The model under review builds one solid part; all positions refer to its coordinate system, in mm. Face numbers are marked on the shaded views. A direction names the side the tool comes from. Round coordinates to 2 decimals unless told otherwise and drop trailing zeros. Order: outer loops, then holes, each group sorted by start corner. A loop starts at its lowest first (then second) coordinate and runs counter-clockwise, first axis right, second up. Notation, with made-up numbers: (46, 83.5) - (66, 83.5) arc R19 ccw to (66, 118.5) - close; hole circle Ø8 at (10, 64.25). An arc over 180 degrees is marked (long way). One line per question, with ' | ' between items. Start each with the question number.
Item 1: Add section C-C on x = -6.5. State how many separate pieces and enclosed holes the cut face has, and give its area (3 significant figures).
Item 2: Add section B-B on y = 8. State the section outline as (x, z) points.
Item 3: Insertion check: pin 1 Ø5 at (y, z) = (36.5, 5) entering from +X; pin 2 Ø6 at (x, z) = (20.98, -7.33) entering from +Y; pin 3 Ø12 at (x, z) = (14.5, 20) entering from +Y; pin 4 Ø16 at (x, y) = (3.5, 17.5) entering from +Z. Each pin has a flat end and moves straight along its axis. Give the tip position at first contact, or say it passes through.
Item 4: Tool access review of the marked faces 4, 5 and 6: name each direction out of +Z, -Z, +X, -X, +Y, -Y from which nothing blocks a thin tool from reaching the whole face with its end or side.
Item 5: For L1, parallel to Z at x = 0, y = 46; L2, parallel to X at y = 31, z = 4; L3, parallel to Y at x = -2, z = -19.5, list the stretches that pass through material, from the lowest coordinate up. Write a range as [from, to].
Item 6: Add section A-A on y = 49. State the section outline as (x, z) points (1 decimal).
Item 7: Draft analysis for pull direction Z (two halves, no side actions). For the marked faces 1, 2 and 3, state which applies: +Z half, -Z half, draft (parallel to the pull), parting line (faces both ways), or undercut.
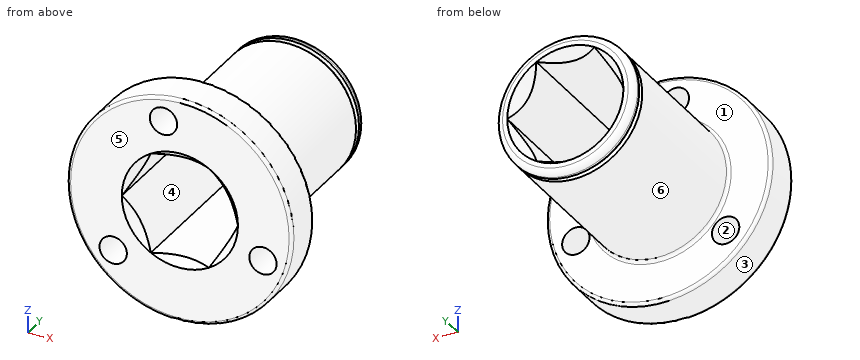
from build123d import *

# Parameters (mm, degrees)
SKETCH2_R                = 28.3845
BOSS_EXTRUDE1_DEPTH      = 10.16
SKETCH3_R                = 17.4625
BOSS_EXTRUDE2_DEPTH      = 44.831
CUT_EXTRUDE1_DEPTH       = 1
CUT_EXTRUDE1_DEPTH_BACK  = 55.991
F_5_16_24_TAPPED_HOLE2_D = 6.9088
SKETCH10_W               = 1.0668
SKETCH10_H               = 1.4224
FILLET1_R                = 1.5875
FILLET2_R                = 0.79375


with BuildPart() as part:
    # Sketch2 → Boss-Extrude1 (new body)
    with BuildSketch(Plane(origin=(0, 0, 0), x_dir=(1, 0, 0), z_dir=(0, 1, 0))):
        Circle(SKETCH2_R)
    extrude(amount=BOSS_EXTRUDE1_DEPTH)

    # Sketch3 → Boss-Extrude2 (add)
    with BuildSketch(Plane(origin=(0, 10.16, 0), x_dir=(1, 0, 0), z_dir=(0, 1, 0))):
        Circle(SKETCH3_R)
    extrude(amount=BOSS_EXTRUDE2_DEPTH)

    # Sketch4 → Cut-Extrude1 (cut, two sides)
    with BuildSketch(Plane(origin=(0, 54.991, 0), x_dir=(1, 0, 0), z_dir=(0, 1, 0))) as cut_extrude1_sk:
        Polygon((14.664696837, 0), (7.332348419, 12.7), (-7.332348419, 12.7), (-14.664696837, 0), (-7.332348419, -12.7), (7.332348419, -12.7), align=None)
    extrude(amount=CUT_EXTRUDE1_DEPTH, mode=Mode.SUBTRACT)
    extrude(cut_extrude1_sk.sketch, amount=-CUT_EXTRUDE1_DEPTH_BACK, mode=Mode.SUBTRACT)

    # 5/16-24 Tapped Hole2 (through all)
    with Locations(Plane(origin=(0, 0, 0), x_dir=(-1, 0, 0), z_dir=(0, -1, 0))):
        with Locations((4.138562858, -21.83627538), (16.841487774, 14.50223826), (-20.980050632, 7.33403712)):
            Hole(F_5_16_24_TAPPED_HOLE2_D / 2)

    # Sketch10 → Cut-Revolve1 (revolve, cut)
    with BuildSketch(Plane.XY):
        Polygon((14.664696837, 54.991), (0, 29.591), (0, 54.991), align=None)
        Polygon((14.664696837, 0), (0, 14.664696837), (0, 0), align=None)
        with Locations((16.9291, 51.9938)):
            Rectangle(SKETCH10_W, SKETCH10_H)
    revolve(axis=Axis((0, 0, 0), (0, 1, 0)), mode=Mode.SUBTRACT)

    # Fillet1
    fillet1_edges = [part.edges().sort_by_distance(p)[0] for p in [
        (-17.4625, 54.991, 0),
    ]]
    fillet(fillet1_edges, radius=FILLET1_R)

    # Fillet2
    fillet2_edges = [part.edges().sort_by_distance(p)[0] for p in [
        (-28.3845, 0, 0),
        (-28.3845, 10.16, 0),
        (-17.4625, 10.16, 0),
    ]]
    fillet(fillet2_edges, radius=FILLET2_R)


solid = part.part
Determined:
1) separate pieces: 3 | enclosed holes: 0 | area: 561 mm2
2) outline: circle Ø56.77 at (0, 0); hole circle Ø6.91 at (-16.84, -14.5); hole (-14.66, 0) - (-7.33, -12.7) - (7.33, -12.7) - (14.66, 0) - (7.33, 12.7) - (-7.33, 12.7) - close; hole circle Ø6.91 at (-4.14, 21.84); hole circle Ø6.91 at (20.98, -7.33)
3) pin 1: x = 17.28 | pin 2: through | pin 3: y = 10.16 | pin 4: z = 28.26
4) face 4: +Y, -Y | face 5: +Z, -Z, +X, -X, -Y | face 6: +Y
5) L1: [-17.46, -12.7], [12.7, 17.46] | L2: [-17, -12.36], [12.36, 17] | L3: [0, 10.16]
6) outline: circle Ø34.9 at (0, 0); hole (-14.7, 0) - (-7.3, -12.7) - (7.3, -12.7) - (14.7, 0) - (7.3, 12.7) - (-7.3, 12.7) - close
7) face 1: draft | face 2: undercut | face 3: parting line
